Job drawing, mm, ordinate dimensions from the low corner. One solid piece. A direction names the side the tool comes from. Coordinates: 2 decimals unless noted, no trailing zeros. Loops run counter-clockwise (first coordinate to the right, second up) from the corner with the lowest first, then second, coordinate; pieces in that order, holes last. Notation, with made-up numbers: (55, 86.25) - (59, 86.25) arc R17 ccw to (59, 109.25) - close; hole circle Ø1 at (-10, 14). An arc over 180 degrees is marked (long way). One line per question, with ' | ' between items. Start each with the question number.
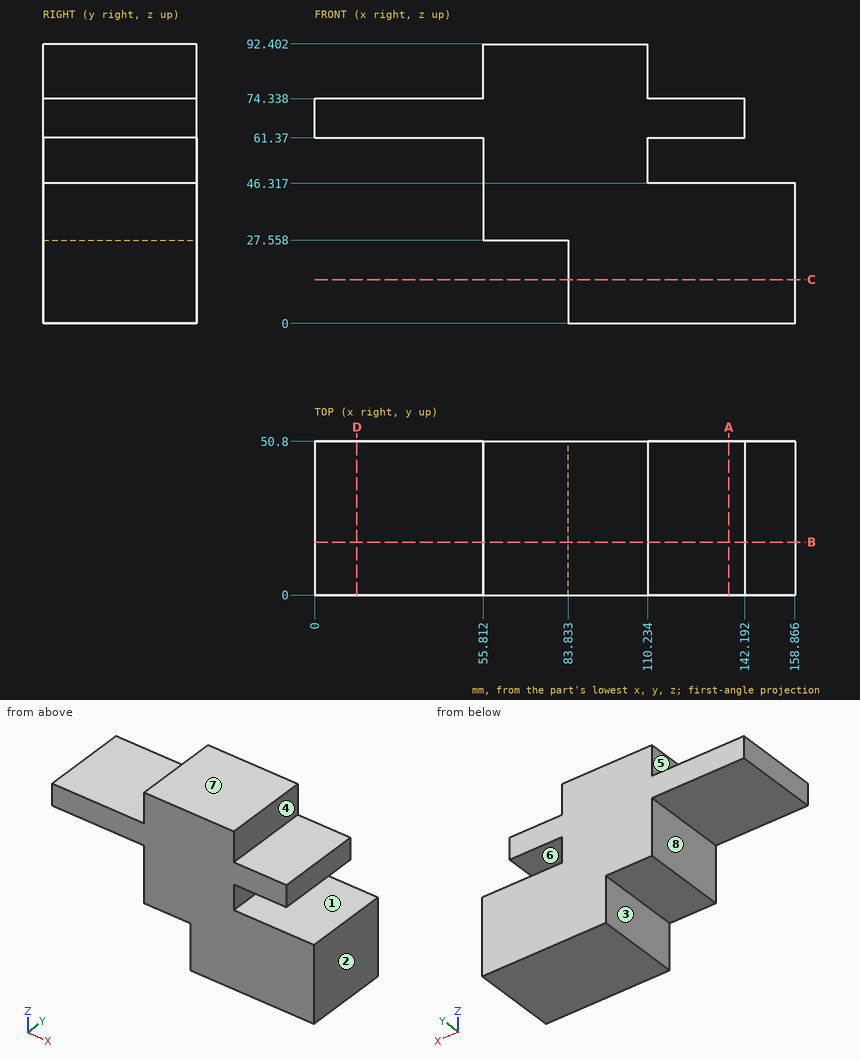
1) Band-saw the part on B-B on y = 17.5. List the corners of the cut face in (x, z).
2) Mould opens along Z. For the marked faces 6, 7 and 8 say: +Z half, -Z half, draft (parallel to the pull), parting line (faces both ways), or undercut.
3) Pin check, flat tips, straight feed: pin 1 Ø16 at (x, y) = (132.5, 15.5) entering from +Z; pin 2 Ø22 at (y, z) = (17, 15.5) entering from -X; pin 3 Ø3 at (y, z) = (20, 67.5) entering from +X. Stop position of each tip, or through.
4) Wall check: line 1 along Z through (x, y) = (129, 30); line 2 along X through (y, z) = (24, 7); line 3 along Z through (x, y) = (27.5, 29). Give the ranges that are in metal, low to high. Write a range as [from, to].
5) Band-saw the part on D-D on x = 14. List the corners of the cut face in (y, z), then the cut area to 3 significant figures.
6) Band-saw the part on A-A on x = 137. List the corners of the cut face in (y, z).
7) Tool access for the marked faces 1, 2, 3, 4 and 5: list every direction of +Z, -Z, +X, -X, +Y, -Y with a clear straight run to the whole face (end or side of a thin tool).
8) Band-saw the part on C-C on z = 14.5. List the corners of the cut face in (x, y), then the cut area to 3 significant figures.
Values found:
1) outline: (0, 61.37) - (55.81, 61.37) - (55.81, 27.56) - (83.83, 27.56) - (83.83, 0) - (158.87, 0) - (158.87, 46.32) - (110.23, 46.32) - (110.23, 61.37) - (142.19, 61.37) - (142.19, 74.34) - (110.23, 74.34) - (110.23, 92.4) - (55.81, 92.4) - (55.81, 74.34) - (0, 74.34) - close
2) face 6: undercut | face 7: +Z half | face 8: draft
3) pin 1: z = 74.34 | pin 2: x = 83.83 | pin 3: x = 142.19
4) line 1: [0, 46.32], [61.37, 74.34] | line 2: [83.83, 158.87] | line 3: [61.37, 74.34]
5) outline: (0, 61.37) - (50.8, 61.37) - (50.8, 74.34) - (0, 74.34) - close | area: 659 mm²
6) outline: (0, 0) - (50.8, 0) - (50.8, 46.32) - (0, 46.32) - close; (0, 61.37) - (50.8, 61.37) - (50.8, 74.34) - (0, 74.34) - close
7) face 1: +X, +Y, -Y | face 2: +Z, -Z, +X, +Y, -Y | face 3: -Z, -X, +Y, -Y | face 4: +Z, +X, +Y, -Y | face 5: +Z, -X, +Y, -Y
8) outline: (83.83, 0) - (158.87, 0) - (158.87, 50.8) - (83.83, 50.8) - close | area: 3,810 mm²
